Part print with two shaded views. Sizes in mm from the minimum x, y, z corner. Give positions to 0.01 mm unless a question says otherwise; leave off trailing zeros. Write each loop counter-clockwise with the first axis right and the second up, starting at its lowest first coordinate (ties: lowest second). Pieces come first, ordered by that corner, then holes.
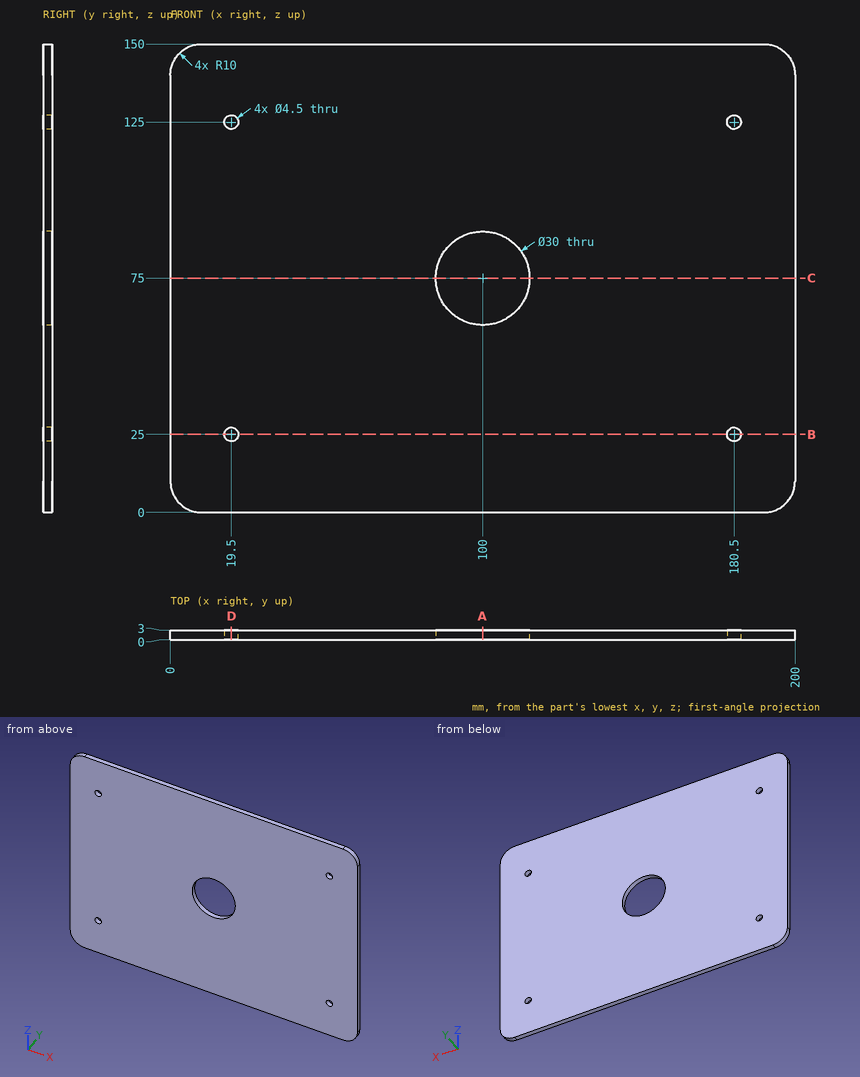
(1) Saw through at C-C, the plane z = 75. List the corners of the cut face in (x, y), plus the area to 3 significant figures.
(2) Saw through at B-B, the plane z = 25. List the corners of the cut face in (x, y).
(3) Saw through at A-A, the plane x = 100. List the corners of the cut face in (y, z), plus the area to 3 significant figures.
(4) Saw through at D-D, the plane x = 19.5. List the corners of the cut face in (y, z), plus the area to 3 significant figures.
(5) Probe line 1 (X direction, y = 0.6, z = 25); line 2 (Z direction, x = 180.5, y = 1.95); line 3 (X direction, y = 1.65, z = 75). List the from-to ranges inside material, lowest first.
Computed values:
1. outline: (0, 0) - (85, 0) - (85, 3) - (0, 3) - close; (115, 0) - (200, 0) - (200, 3) - (115, 3) - close
1. area: 510 mm2
2. outline: (0, 0) - (17.25, 0) - (17.25, 3) - (0, 3) - close; (21.75, 0) - (178.25, 0) - (178.25, 3) - (21.75, 3) - close; (182.75, 0) - (200, 0) - (200, 3) - (182.75, 3) - close
3. outline: (0, 0) - (3, 0) - (3, 60) - (0, 60) - close; (0, 90) - (3, 90) - (3, 150) - (0, 150) - close
3. area: 360 mm2
4. outline: (0, 0) - (3, 0) - (3, 22.75) - (0, 22.75) - close; (0, 27.25) - (3, 27.25) - (3, 122.75) - (0, 122.75) - close; (0, 127.25) - (3, 127.25) - (3, 150) - (0, 150) - close
4. area: 423 mm2
5. line 1: x = 0 to 17.25, 21.75 to 178.25, 182.75 to 200
5. line 2: z = 0 to 22.75, 27.25 to 122.75, 127.25 to 150
5. line 3: x = 0 to 85, 115 to 200
